Geometry: final body of the model. Coordinates: model frame, mm. A direction names the side the tool comes from. Round coordinates to 2 decimals unless told otherwise and drop trailing zeros. Loops run counter-clockwise (first coordinate to the right, second up) from the corner with the lowest first, then second, coordinate; pieces in that order, holes last. Notation, with made-up numbers: (-23.5, 76) - (7.5, 76) arc R28 ccw to (7.5, 103) - close; hole circle Ø6 at (88, 32.25). An arc over 180 degrees is marked (long way). Write item = value, one per line. Start each with the question number.
Item 1: Section B-B (z = 10). Return loops of the section in (x, y).
Item 2: Section D-D (x = -7). Return loops of the section in (y, z).
Item 3: Access query for faces 1 (the flat face through (-6, 0, 10)), 2 (the flat face through (-13, -5, 20)). Directions: +Z, -Z, +X, -X, +Y, -Y. A direction counts if a zero-diameter tool reaches every point of the face in a straight line with its end or side. Return the directions, or none.
Item 4: Draft query along X for faces 3 (the flat face through (-5, 4, 10)), 4 (the flat face through (0, -17, 10)), 5 (the flat face through (3.972, -15.773, 9.86)). Return one class per face: pulls with the +X half, pulls with the -X half, needs draft (parallel to the pull), parting line crosses it, or undercut.
Item 5: Section C-C (y = -6). Return loops of the section in (x, z), plus the area to 3 significant figures.
Item 6: Line query: line 1 (Y direction, x = -3.5, z = 2); line 2 (X direction, y = -26, z = 16); line 3 (X direction, y = -11.5, z = 2). Output: solid intervals per line, ascending. Write a range as from..to.
Item 7: Section A-A (y = -24). Return loops of the section in (x, z), plus the area to 3 significant figures.
Item 8: First-contact query: pin 1 (1.5 mm diameter, centred on y = 14.5, z = 2, fed in from -X); pin 2 (6 mm diameter, centred on x = 0.5, z = 9.5, fed in from +Y); pin 3 (6 mm diameter, centred on y = -19.5, z = 5.5, fed in from -X). Flat tips, straight axial feed; report the tip coordinate or a pass-through.
from build123d import *

# Parameters (mm, degrees)
PAD_DEPTH = 20


with BuildPart() as part:
    # Sketch → Pad (new body)
    with BuildSketch(Plane.XY):
        with BuildLine():
            Line((0, 0), (0, -35))
            Line((0, -35), (2, -35))
            Line((2, -35), (6, 4))
            Line((6, 4), (-15.443946, 4))
            ThreePointArc((-29.038563, 12.660726), (-23.50344, 6.349128), (-15.443946, 4))
            Line((-29.038563, 12.660726), (-34.326153, 24))
            Line((-34.326153, 24), (-35.326153, 24))
            Line((-14, -35), (-35.326153, 24))
            Line((-14, -35), (-12, -35))
            Line((-12, -35), (-12, 0))
            Line((-12, 0), (0, 0))
        make_face()
    extrude(amount=PAD_DEPTH)


solid = part.part
Taken from the geometry:
q1.outline = (-35.33, 24) - (-14, -35) - (-12, -35) - (-12, 0) - (0, 0) - (0, -35) - (2, -35) - (6, 4) - (-15.44, 4) arc R15 cw to (-29.04, 12.66) - (-34.33, 24) - close
q2.outline = (0, 0) - (4, 0) - (4, 20) - (0, 20) - close
q3.face_1 = +Z, -Z, -Y
q3.face_2 = +Z, +X, -X, +Y, -Y
q4.face_3 = needs draft
q4.face_4 = undercut
q4.face_5 = pulls with the +X half
q5.outline = (-24.48, 0) - (-12, 0) - (-12, 20) - (-24.48, 20) - close; (0, 0) - (4.97, 0) - (4.97, 20) - (0, 20) - close
q5.area = 349 mm^2
q6.line_1 = 0..4
q6.line_2 = -17.25..-12, 0..2.92
q6.line_3 = -22.49..-12, 0..4.41
q7.outline = (-17.98, 0) - (-12, 0) - (-12, 20) - (-17.98, 20) - close; (0, 0) - (3.13, 0) - (3.13, 20) - (0, 20) - close
q7.area = 182 mm^2
q8.pin_1 = -32.16
q8.pin_2 = 4
q8.pin_3 = -20.69
